The model under review builds one solid part; all positions refer to its coordinate system, in mm. A direction names the side the tool comes from. Coordinates: 2 decimals unless noted, no trailing zeros. Order: outer loops, then holes, each group sorted by start corner. A loop starts at its lowest first (then second) coordinate and runs counter-clockwise, first axis right, second up. Notation, with made-up numbers: (-37.75, 4) -> (-26.75, 4) arc R26 ccw to (-26.75, 34) -> close; hole circle Ø8 at (43.5, 47). An arc over 180 degrees is marked (long way). Use one line per item in the form item = value. Start each with the question number.
(1) Take a section at A-A (z = 6). State the section outline as (x, y) points, then the cut area to 3 significant figures.
(2) Take a section at D-D (z = -8.5). State the section outline as (x, y) points, then the cut area to 3 significant figures.
(3) Take a section at C-C (x = -8). State the section outline as (y, z) points, then the cut area to 3 significant figures.
(4) Take a section at B-B (y = -121.5). State the section outline as (x, z) points, then the cut area to 4 significant figures.
(5) Insertion check: pin 1 Ø22.5 at (x, z) = (-114.5, -9) entering from -Y; pin 2 Ø3 at (y, z) = (-39.5, 9.5) entering from +X; pin 3 Ø1 at (x, z) = (-187, -12) entering from -Y. Each pin has a flat end and moves straight along its axis. Give the tip position at first contact, or say it passes through.
(6) For faces 5 (the flat face through (-190, -99, 0)), 6 (the flat face through (-230.8, -190.6, -0.3)), 7 (the flat face through (-190.3, -68.9, -22.5)), 8 (the flat face through (-215, -87, 0)), 9 (the flat face through (-189.01, -187.61, -0.32)), list the 3-axis set-ups (+Z, -Z, +X, -X, +Y, -Y) from which the entire face can be reached by the end or side of a thin tool; tool diameter is ignored.
(7) Wall thickness on line 1 along X through (y, z) = (-44.5, 7.5); line 2 along Y through (x, z) = (-83, 8); line 3 along Y through (x, z) = (-200, -15): over which ranges is each line inside the solid? List them lowest first.
(8) Mouldability with a two-part tool opening along Y and no side actions: class faces 1 (the cylindrical face through (-203.53, -13.33, 0.32)), 2 (the cylindrical face through (-0.56, 11.923, -3.755)), 3 (the flat face through (40, 0, 0)), 4 (the cylindrical face through (-172.129, -29.982, -0.315)) as +Y half, -Y half, draft (parallel to the pull), parting line (faces both ways), or undercut.
Autodesk Inventor part; units mm, degrees
ref_plane "YZ Plane" through (0, 0, 0) normal (1, 0, 0) x (0, 1, 0)
ref_plane "XZ Plane" through (0, 0, 0) normal (0, 1, 0) x (-1, 0, 0)
ref_plane "XY Plane" through (0, 0, 0) normal (0, 0, 1) x (1, 0, 0)
sketch "Sketch1" plane through (0, 0, 0) normal (1, 0, 0) x (0, 1, 0)
  circle A0 centre (0, 0) radius 12.5
  dimension "d0" = 25
extrude "Extrusion1" add sketch "Sketch1" along normal mid plane 80
sketch "Sketch2" plane through (0, 0, 0) normal (0, 0, 1) x (1, 0, 0)
  line L0 (-40, 12.5) -> (-40, -12.5)
  line L1 (-40, 12.5) -> (-190, 12.5)
  line L2 (-40, -12.5) -> (-165, -12.5)
  circle A0 centre (-190, -12.5) radius 25
  line L3 (-215, -12.5) -> (-215, -164.1266)
  line L4 (-190, -37.5) -> (-190, -162.5)
  line L5 (-190, -162.5) -> (-165.4254, -179.7073)
  line L6 (-190, -162.5) -> (-160, -162.5) construction
  line L7 (-165.4254, -179.7073) -> (-176.897, -196.0903)
  line L8 (-176.897, -196.0903) -> (-201.4715, -178.883)
  line L9 (-201.4715, -178.883) -> (-224.4529, -198.1667)
  line L10 (-224.4529, -198.1667) -> (-237.3086, -182.8458)
  line L11 (-237.3086, -182.8458) -> (-215, -164.1266)
  point P0 (0, 0)
  point P1 (-165, -12.5)
  dimension "d3" = 150
  dimension "d4" = 125
extrude "Extrusion2" add sketch "Sketch2" along normal mid plane 45
sketch "Sketch3" plane through (0, 0, -22.5) normal (0, 0, -1) x (-1, 0, 0)
  circle A0 centre (191.1384, -11.6978) radius 12.5
  point P0 (0, 0)
hole "Hole1" at (-191.1384, -11.6978, -22.5) direction (0, 0, 1) diameter 25 depth 45
properties part number "Hand 4"
Findings:
q1.outline = (-237.31, -182.85) -> (-224.45, -198.17) -> (-201.47, -178.88) -> (-176.9, -196.09) -> (-165.43, -179.71) -> (-190, -162.5) -> (-190, -37.5) arc R25 ccw to (-165, -12.5) -> (-40, -12.5) -> (-40, -10.97) -> (40, -10.97) -> (40, 10.97) -> (-40, 10.97) -> (-40, 12.5) -> (-190, 12.5) arc R25 ccw to (-215, -12.5) -> (-215, -164.13) -> close; hole circle Ø25 at (-191.14, -11.7)
q1.area = 11,200 mm²
q2.outline = (-237.31, -182.85) -> (-224.45, -198.17) -> (-201.47, -178.88) -> (-176.9, -196.09) -> (-165.43, -179.71) -> (-190, -162.5) -> (-190, -37.5) arc R25 ccw to (-165, -12.5) -> (-40, -12.5) -> (-40, -9.17) -> (40, -9.17) -> (40, 9.17) -> (-40, 9.17) -> (-40, 12.5) -> (-190, 12.5) arc R25 ccw to (-215, -12.5) -> (-215, -164.13) -> close; hole circle Ø25 at (-191.14, -11.7)
q2.area = 10,900 mm²
q3.outline = circle Ø25 at (0, 0)
q3.area = 491 mm²
q4.outline = (-215, -22.5) -> (-190, -22.5) -> (-190, 22.5) -> (-215, 22.5) -> close
q4.area = 1,125 mm²
q5.pin_1 = -12.5
q5.pin_2 = -190
q5.pin_3 = -189.37
q6.face_5 = +Z, -Z, +X
q6.face_6 = +Z, -Z, -X, -Y
q6.face_7 = -Z, +X, -X, +Y, -Y
q6.face_8 = +Z, -Z, -X, +Y
q6.face_9 = +Z, -Z, -Y
q7.line_1 = -215 to -190
q7.line_2 = -12.5 to 12.5
q7.line_3 = -179.91 to -20.51, -2.88 to 10.41
q8.face_1 = undercut
q8.face_2 = parting line
q8.face_3 = draft
q8.face_4 = undercut
